Could you check a few things on this model? Use its own coordinates, in mm. Coordinates: 2 decimals unless noted, no trailing zeros. Loops run counter-clockwise (first coordinate to the right, second up) from the corner with the lowest first, then second, coordinate; pieces in that order, holes last.
Autodesk Inventor part; units mm, degrees
ref_plane "YZ Plane" through (0, 0, 0) normal (1, 0, 0) x (0, 1, 0)
ref_plane "XZ Plane" through (0, 0, 0) normal (0, 1, 0) x (-1, 0, 0)
ref_plane "XY Plane" through (0, 0, 0) normal (0, 0, 1) x (1, 0, 0)
sketch "Sketch1" plane through (0, 0, 0) normal (0, 0, 1) x (1, 0, 0)
  line L0 (-177.8, 127) -> (177.8, 127)
  line L1 (177.8, 127) -> (177.8, -127)
  line L2 (177.8, -127) -> (-177.8, -127)
  line L3 (-177.8, -127) -> (-177.8, 127)
  line L4 (-88.8998, 127) -> (-88.8998, -127)
  line L5 (88.9077, 127) -> (88.9077, -127)
  line L6 (-88.8998, 0) -> (88.9077, 0)
  point P0 (0, 0)
  dimension "d0" = 355.6
  dimension "d1" = 254
extrude "Extrusion1" add sketch "Sketch1" along normal blind 1.5875 contours L0 L4 L2 L3 | L0 L5 L6 L4 | L0 L1 L2 L5
fillet "Fillet1" radius 3.175 1 edges at (177.8, 127, 0.7937)
fillet "Fillet2" radius 3.175 1 edges at (177.8, -127, 0.7937)
fillet "Fillet3" radius 3.175 1 edges at (-88.8998, -127, 0.7937)
fillet "Fillet4" radius 3.175 1 edges at (-88.8998, 0, 0.7937)
fillet "Fillet5" radius 3.175 1 edges at (-177.8, -127, 0.7937)
fillet "Fillet6" radius 3.175 1 edges at (-177.8, 127, 0.7937)
fillet "Fillet7" radius 3.175 1 edges at (88.9077, -127, 0.7937)
fillet "Fillet8" radius 3.175 1 edges at (88.9077, 0, 0.7937)
properties part number "Blocker"
1) Imagine slicing it at C-C on x = 12. List the corners of the cut face in (y, z) for me, plus the area to 3 significant figures.
2) Imagine slicing it at A-A on y = -32.5. List the corners of the cut face in (x, z) for me.
3) If I drill on L1, parallel to X at y = -38.5, z = 0.5; L2, parallel to Y at x = -9.5, z = 1.35; L3, parallel to X at y = -2, z = 0.95, over which ranges is the centre line in solid material (lowest first)?
4) Imagine slicing it at B-B on z = 0.25. List the corners of the cut face in (x, y) for me (3 decimals), plus the area to 3 significant figures.
Solved:
1. outline: (0, 0) - (127, 0) - (127, 1.59) - (0, 1.59) - close
1. area: 202 mm2
2. outline: (-177.8, 0) - (-88.9, 0) - (-88.9, 1.59) - (-177.8, 1.59) - close; (88.91, 0) - (177.8, 0) - (177.8, 1.59) - (88.91, 1.59) - close
3. L1: x = -177.8 to -88.9, 88.91 to 177.8
3. L2: y = 0 to 127
3. L3: x = -177.8 to -88.67, 88.68 to 177.8
4. outline: (-177.8, -123.825) arc R3.175 ccw to (-174.625, -127) - (-92.075, -127) arc R3.175 ccw to (-88.9, -123.825) - (-88.9, -3.175) arc R3.175 cw to (-85.725, 0) - (85.733, 0) arc R3.175 cw to (88.908, -3.175) - (88.908, -123.825) arc R3.175 ccw to (92.083, -127) - (174.625, -127) arc R3.175 ccw to (177.8, -123.825) - (177.8, 123.825) arc R3.175 ccw to (174.625, 127) - (-174.625, 127) arc R3.175 ccw to (-177.8, 123.825) - close
4. area: 67,700 mm2
